The model under review builds one solid part; all positions refer to its coordinate system, in mm. A direction names the side the tool comes from. Round coordinates to 2 decimals unless told otherwise and drop trailing zeros. Order: outer loops, then holes, each group sorted by start corner. A loop starts at its lowest first (then second) coordinate and runs counter-clockwise, first axis right, second up.
1) Clearance check with flat-ended pins moving along their axes: P1, Ø5, axis at y = 12, z = 40, coming from the +X side; P2, Ø3.5, axis at y = 22.12, z = 71.15, coming from the -X side; P3, Ø6.5, axis at x = -18, z = 40, coming from the +Y side. State where each tip first meets the part, or that it passes through.
2) Mouldability with a two-part tool opening along Y and no side actions: class faces 4 (the face through (34, 14, 39)), 5 (the face through (32, 17, 40)), 6 (the face through (-31.97, 23.81, 9.92)), 7 (the face through (0, -4, 39)) as pulls with the +Y half, pulls with the -Y half, needs draft (parallel to the pull), parting line crosses it, or undercut.
3) Consider section C-C (z = 40). Give the boundary of the cut face in (x, y).
4) Consider section A-A (y = 12). Give the boundary of the cut face in (x, z), then the cut area to 3 significant figures.
5) Consider section B-B (x = -9). Give the boundary of the cut face in (y, z).
6) Consider section D-D (y = 2.5). Give the boundary of the cut face in (x, z).
7) To check wall thickness, follow L1, parallel to Z at x = -9, y = -1.85; L2, parallel to Z at x = -18, y = -1.1; L3, parallel to X at y = 11, z = 30.5. State the ranges of each line that lie inside material, in increasing order.
8) Machinability: for faces 1 (the face through (32.028, 26.765, 69.469)), 2 (the face through (0, 0, 39)), 3 (the face through (16, -2, 38.5)), which of the approach directions +Z, -Z, +X, -X, +Y, -Y give a long, thin tool a straight path to every point of the face, cutting with its end or side? Answer none if there is none.
from build123d import *

# Parameters (mm, degrees)
SM_BASE_FLANGE_1_DEPTH   = 80
CUT_EXTRUDE_3_DEPTH      = 109.411254028
CUT_EXTRUDE_3_DEPTH_BACK = 109.411254028
SKETCH_6_R               = 48
SKETCH_6_R_2             = 2
FILLET_1_R               = 5
SKETCH_9_R               = 2.5
CUT_EXTRUDE_4_DEPTH      = 93.287593966


# Sheet-metal steps are written as plain solids
with BuildPart() as part:
    # Sketch 1 → Базовая кромка1 (new body)
    with BuildSketch(Plane.XY):
        with BuildLine():
            Line((-30, 27), (-30, 1))
            ThreePointArc((-30, 1), (-29.707106781, 0.292893219), (-29, 0))
            Line((-29, 0), (29, 0))
            ThreePointArc((29, 0), (29.707106781, 0.292893219), (30, 1))
            Line((30, 1), (30, 27))
            Line((30, 27), (34, 27))
            Line((34, 27), (34, 1))
            ThreePointArc((34, 1), (32.535533906, -2.535533906), (29, -4))
            Line((29, -4), (-29, -4))
            ThreePointArc((-29, -4), (-32.535533906, -2.535533906), (-34, 1))
            Line((-34, 1), (-34, 27))
            Line((-34, 27), (-30, 27))
        make_face()
    extrude(amount=SM_BASE_FLANGE_1_DEPTH)

    # Эскиз6 → Вырез-Вытянуть3 (cut, two sides: drawn at the far end of the back side and taken through both)
    with BuildSketch(Plane.ZY.offset(34).offset(-CUT_EXTRUDE_3_DEPTH_BACK)):
        with Locations((40, 65)):
            Circle(SKETCH_6_R)
        with Locations((40, 12)):
            Circle(SKETCH_6_R_2)
        with Locations((8.847381628, 22.122099298)):
            Circle(SKETCH_6_R_2)
        with Locations((71.152618372, 22.122099298)):
            Circle(SKETCH_6_R_2)
    extrude(amount=CUT_EXTRUDE_3_DEPTH + CUT_EXTRUDE_3_DEPTH_BACK, mode=Mode.SUBTRACT)

    # Скругление1
    fillet_1_edges = [part.edges().sort_by_distance(p)[0] for p in [
        (32, 27, 10.674243403),
        (32, 27, 69.325756597),
        (-32, 27, 10.674243403),
        (-32, 27, 69.325756597),
    ]]
    fillet(fillet_1_edges, radius=FILLET_1_R)

    # Эскиз9 → Вырез-Вытянуть4 (cut, through all)
    with BuildSketch(Plane.XZ.offset(4)):
        with Locations((-18, 40)):
            Circle(SKETCH_9_R)
        with Locations((-9, 55.588457268)):
            Circle(SKETCH_9_R)
        with Locations((9, 55.588457268)):
            Circle(SKETCH_9_R)
        with Locations((18, 40)):
            Circle(SKETCH_9_R)
        with Locations((9, 24.411542732)):
            Circle(SKETCH_9_R)
        with Locations((-9, 24.411542732)):
            Circle(SKETCH_9_R)
    extrude(amount=-CUT_EXTRUDE_4_DEPTH, mode=Mode.SUBTRACT)


solid = part.part
Answer below:
1. P1: stops at x = 34
1. P2: passes through
1. P3: stops at y = 0
2. face 4: needs draft
2. face 5: pulls with the +Y half
2. face 6: undercut
2. face 7: pulls with the -Y half
3. outline: (-34, 1) arc R5 ccw to (-29, -4) - (-20.5, -4) - (-20.5, 0) - (-29, 0) arc R1 cw to (-30, 1) - (-30, 10) - (-34, 10) - close; (-34, 14) - (-30, 14) - (-30, 17) - (-34, 17) - close; (-15.5, -4) - (15.5, -4) - (15.5, 0) - (-15.5, 0) - close; (20.5, -4) - (29, -4) arc R5 ccw to (34, 1) - (34, 10) - (30, 10) - (30, 1) arc R1 cw to (29, 0) - (20.5, 0) - close; (30, 14) - (34, 14) - (34, 17) - (30, 17) - close
4. outline: (-34, 0) - (-30, 0) - (-30, 38) - (-34, 38) - close; (-34, 42) - (-30, 42) - (-30, 80) - (-34, 80) - close; (30, 0) - (34, 0) - (34, 38) - (30, 38) - close; (30, 42) - (34, 42) - (34, 80) - (30, 80) - close
4. area: 608 mm2
5. outline: (-4, 0) - (0, 0) - (0, 21.91) - (-4, 21.91) - close; (-4, 26.91) - (0, 26.91) - (0, 53.09) - (-4, 53.09) - close; (-4, 58.09) - (0, 58.09) - (0, 80) - (-4, 80) - close
6. outline: (-34, 0) - (-30, 0) - (-30, 80) - (-34, 80) - close; (30, 0) - (34, 0) - (34, 80) - (30, 80) - close
7. L1: z = 0 to 21.91, 26.91 to 53.09, 58.09 to 80
7. L2: z = 0 to 37.5, 42.5 to 80
7. L3: x = -34 to -30, 30 to 34
8. face 1: +X, -X, +Y
8. face 2: +Z, -Z, +Y
8. face 3: +Y, -Y
